Source: CAD feature listing. Evaluate the final solid. Frame: model axes, mm. A direction names the side the tool comes from. Give positions to 0.01 mm unless a question says otherwise; leave off trailing zeros. Write each loop counter-clockwise with the first axis right and the second up, starting at its lowest first coordinate (ties: lowest second). Pieces come first, ordered by that corner, then holes. Notation, with made-up numbers: (-5.75, 11) -> (52.25, 11) arc R24 cw to (52.25, 42) -> close; hole circle Ø11 at (-29.5, 43). An arc over 180 degrees is marked (long way). Answer as a JSON object with one key per item and string values. Group by question number.
Item 1: Section query A-A on y = 0. Return the cut outline in (x, z).
Item 2: Section query D-D on x = 26. Return the cut outline in (y, z).
Item 3: Access query for faces 4 (the face through (-62.861, -6.324, 4.032)), 5 (the face through (9.44, -6.324, 4.032)), 6 (the face through (19, 5.7, 0)). Directions: +Z, -Z, +X, -X, +Y, -Y. A direction counts if a zero-diameter tool reaches every point of the face in a straight line with its end or side. Return the directions, or none.
Item 4: First-contact query: pin 1 Ø0.6 at (x, y) = (-35.5, 8) entering from -Z; pin 2 Ø4 at (x, z) = (1.5, 1.5) entering from +Y; pin 3 Ø1.8 at (x, z) = (-41.5, 1) entering from +Y. Flat tips, straight axial feed; report the tip coordinate or a pass-through.
Item 5: Pull-direction query (Z, two-part tool) for faces 1 (the face through (-34.954, -8.923, -1.172)), 2 (the face through (36.808, 0, 0)), 3 (the face through (31.808, 6.413, -0.055)); classes: pulls with the +Z half, pulls with the -Z half, needs draft (parallel to the pull), parting line crosses it, or undercut.
Item 6: Ray query, probe 1 along Z at (x, y) = (-32, 5); probe 2 along X at (y, z) = (-3.5, -7.5); probe 3 along X at (y, z) = (7.75, 6.5). Return the intervals inside material, ascending. Write a range as from..to.
Item 7: Section query C-C on x = 0.5. Return the cut outline in (y, z), plus the area to 3 significant figures.
Item 8: Section query B-B on z = 0. Return the cut outline in (x, y).
from build123d import *

# Parameters (mm, degrees)
CUT_EXTRUDE1_DEPTH = 2.5
CUT_EXTRUDE2_DEPTH = 1.8
CHAMFER1_SIZE      = 0.5


with BuildPart() as part:
    # Sketch1 → Revolve1 (revolve)
    with BuildSketch(Plane.XY, mode=Mode.PRIVATE) as revolve1_sk:
        Polygon((-69.191650854, 0), (-69.191650854, 7.5), (-57.191650854, 7.5), (-57.191650854, 12), (-52.191650854, 12), (-52.191650854, 9), (-18.191650854, 9), (-18.191650854, 7.5), (36.808349146, 7.5), (36.808349146, 0), align=None)
    revolve(revolve1_sk.sketch.rotate(Axis((-89.707779886, 0, 0), (1, 0, 0)), 90), axis=Axis((-89.707779886, 0, 0), (1, 0, 0)))

    # Sketch2 → Cut-Extrude1 (cut)
    with BuildSketch(Plane(origin=(0, 9, 0), x_dir=(1, 0, 0), z_dir=(0, 1, 0))):
        with BuildLine():
            Line((-44.191650854, 3), (-30.191650854, 3))
            ThreePointArc((-30.191650854, 3), (-27.191650854, 0), (-30.191650854, -3))
            Line((-30.191650854, -3), (-44.191650854, -3))
            ThreePointArc((-44.191650854, -3), (-47.191650854, 0), (-44.191650854, 3))
        make_face()
    extrude(amount=-CUT_EXTRUDE1_DEPTH, mode=Mode.SUBTRACT)

    # Sketch3 → Cut-Extrude2 (cut)
    with BuildSketch(Plane(origin=(0, 7.5, 0), x_dir=(1, 0, 0), z_dir=(0, 1, 0))):
        with BuildLine():
            Line((9.308349146, 2.5), (29.308349146, 2.5))
            ThreePointArc((29.308349146, 2.5), (31.808349146, 0), (29.308349146, -2.5))
            Line((29.308349146, -2.5), (9.308349146, -2.5))
            ThreePointArc((9.308349146, -2.5), (6.808349146, 0), (9.308349146, 2.5))
        make_face()
    extrude(amount=-CUT_EXTRUDE2_DEPTH, mode=Mode.SUBTRACT)

    # Chamfer1
    chamfer1_edges = [part.edges().sort_by_distance(p)[0] for p in [
        (-69.191650854, 0, -7.5),
        (36.808349146, 0, -7.5),
    ]]
    chamfer(chamfer1_edges, length=CHAMFER1_SIZE)


solid = part.part
Worked answers:
{
 "1": {"outline": "(-69.19, -7) -> (-68.69, -7.5) -> (-57.19, -7.5) -> (-57.19, -12) -> (-52.19, -12) -> (-52.19, -9) -> (-18.19, -9) -> (-18.19, -7.5) -> (36.31, -7.5) -> (36.81, -7) -> (36.81, 7) -> (36.31, 7.5) -> (-18.19, 7.5) -> (-18.19, 9) -> (-52.19, 9) -> (-52.19, 12) -> (-57.19, 12) -> (-57.19, 7.5) -> (-68.69, 7.5) -> (-69.19, 7) -> close"},
 "2": {"outline": "(5.7, -2.5) -> (5.7, 2.5) -> (7.07, 2.5) arc R7.5 ccw (long way) to (7.07, -2.5) -> close"},
 "3": {"face 4": "-X", "face 5": "+X", "face 6": "+Y"},
 "4": {"pin 1": "z = -4.66", "pin 2": "y = 7.5", "pin 3": "y = 6.5"},
 "5": {"face 1": "parting line crosses it", "face 2": "needs draft", "face 3": "undercut"},
 "6": {"probe 1": "-7.48..7.48", "probe 2": "-57.19..-18.19", "probe 3": "-57.19..-52.19"},
 "7": {"outline": "circle Ø15 at (0, 0)", "area": "177 mm^2"},
 "8": {"outline": "(-69.19, -7) -> (-68.69, -7.5) -> (-57.19, -7.5) -> (-57.19, -12) -> (-52.19, -12) -> (-52.19, -9) -> (-18.19, -9) -> (-18.19, -7.5) -> (36.31, -7.5) -> (36.81, -7) -> (36.81, 7) -> (36.31, 7.5) -> (31.81, 7.5) -> (31.81, 5.7) -> (6.81, 5.7) -> (6.81, 7.5) -> (-18.19, 7.5) -> (-18.19, 9) -> (-27.19, 9) -> (-27.19, 6.5) -> (-47.19, 6.5) -> (-47.19, 9) -> (-52.19, 9) -> (-52.19, 12) -> (-57.19, 12) -> (-57.19, 7.5) -> (-68.69, 7.5) -> (-69.19, 7) -> close"}
}
